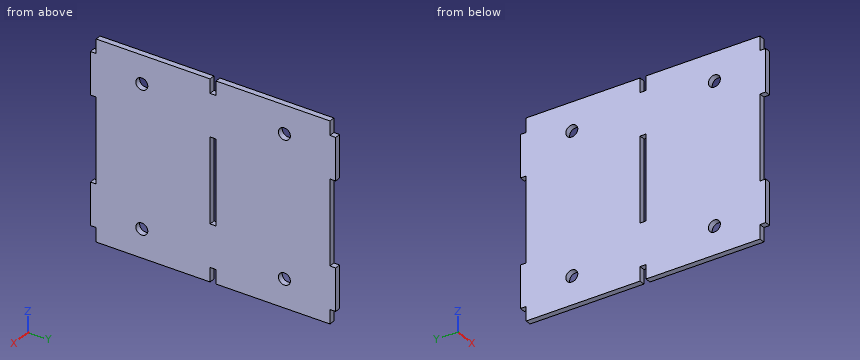
Autodesk Inventor part; units mm, degrees
ref_plane "YZ Plane" through (0, 0, 0) normal (1, 0, 0) x (0, 1, 0)
ref_plane "XZ Plane" through (0, 0, 0) normal (0, 1, 0) x (-1, 0, 0)
ref_plane "XY Plane" through (0, 0, 0) normal (0, 0, 1) x (1, 0, 0)
sketch "Sketch1" plane through (0, 0, 0) normal (1, 0, 0) x (0, 1, 0)
  line L0 (0, 15) -> (0, 0)
  line L1 (0, 15) -> (-2, 15)
  line L2 (-2, 15) -> (-2, 30)
  line L3 (-2, 30) -> (0, 30)
  line L4 (0, 30) -> (0, 35)
  line L5 (0, 35) -> (39.95, 35)
  line L6 (20, 0) -> (0, 0) construction
  line L7 (39.95, 35) -> (39.95, 30)
  line L8 (39.95, 30) -> (42.05, 30)
  line L9 (42.05, 15) -> (39.95, 15)
  line L10 (39.95, 15) -> (39.95, 0)
  line L11 (39.95, 0) -> (20, 0) construction
  line L12 (0, -15) -> (0, 0)
  line L13 (0, -15) -> (-2, -15)
  line L14 (-2, -15) -> (-2, -30)
  line L15 (-2, -30) -> (0, -30)
  line L16 (0, -30) -> (0, -35)
  line L17 (0, -35) -> (39.95, -35)
  line L18 (39.95, -35) -> (39.95, -30)
  line L19 (39.95, -30) -> (42.05, -30)
  line L20 (42.05, -15) -> (39.95, -15)
  line L21 (39.95, -15) -> (39.95, 0)
  line L22 (41, 30) -> (41, -30) construction
  line L23 (82, 15) -> (82, 0)
  line L24 (82, 15) -> (84, 15)
  line L25 (84, 30) -> (82, 30)
  line L26 (82, 30) -> (82, 35)
  line L27 (82, 35) -> (42.05, 35)
  line L28 (42.05, 35) -> (42.05, 30)
  line L29 (42.05, 15) -> (42.05, 0)
  line L30 (42.05, -35) -> (42.05, -30)
  line L31 (42.05, -15) -> (42.05, 0)
  line L32 (82, -15) -> (84, -15)
  line L33 (84, -15) -> (84, -30)
  line L34 (84, -30) -> (82, -30)
  line L35 (82, -30) -> (82, -35)
  line L36 (82, -15) -> (82, 0)
  line L37 (82, -35) -> (42.05, -35)
  line L38 (84, 30) -> (84, 15)
  dimension "d3" = 15
  dimension "d6" = 20
  dimension "d7" = 35
  dimension "d8" = 15
  dimension "d9" = 2
  dimension "d17" = 2.1
  dimension "d23" = 41
extrude "Wyciągnięcie proste1" add sketch "Sketch1" along normal blind 2
sketch "Szkic3" plane through (2, 0, 0) normal (1, 0, 0) x (0, 0, -1)
  line L0 (-25, 16) -> (25, 16) construction
  line L1 (25, 16) -> (25, 66) construction
  line L2 (25, 66) -> (-25, 66) construction
  line L3 (-25, 66) -> (-25, 16) construction
  line L4 (-25, 16) -> (25, 66) construction
  line L5 (25, 16) -> (-25, 66) construction
  line L6 (0, 41) -> (0, 42.05) construction
  line L7 (-15, 42.05) -> (15, 42.05) construction
  line L8 (0, 41) -> (15, 41) construction
  line L9 (15, 42.05) -> (15, 39.95) construction
  circle A0 centre (-25, 66) radius 2.1
  circle A1 centre (25, 66) radius 2.1
  circle A2 centre (25, 16) radius 2.1
  circle A3 centre (-25, 16) radius 2.1
  point P0 (0, 0)
  dimension "d18" = 4.2
  dimension "d19" = 50
  dimension "d20" = 50
extrude "Wyciągnięcie proste2" cut sketch "Szkic3" against normal up to surface (2 mm away)
sketch "Sketch4" plane through (2, 0, 0) normal (1, 0, 0) x (0, 0, -1)
  circle A0 centre (25, 16) radius 2.1
  circle A1 centre (-25, 16) radius 2.1
  circle A2 centre (25, 66) radius 2.1
  circle A3 centre (-25, 66) radius 2.1
  line L0 (-15, 42.05) -> (15, 42.05)
  line L1 (15, 42.05) -> (15, 39.95)
  line L2 (15, 39.95) -> (-15, 39.95)
  line L3 (-15, 39.95) -> (-15, 42.05)
  line L4 (-15, 0) -> (15, 0)
  line L5 (15, 0) -> (15, -2)
  line L6 (15, -2) -> (30, -2)
  line L7 (30, -2) -> (30, 0)
  line L8 (30, 0) -> (35, 0)
  line L9 (35, 0) -> (35, 39.95)
  line L10 (35, 39.95) -> (30, 39.95)
  line L11 (30, 39.95) -> (30, 42.05)
  line L12 (30, 42.05) -> (35, 42.05)
  line L13 (35, 42.05) -> (35, 82)
  line L14 (35, 82) -> (30, 82)
  line L15 (30, 82) -> (30, 84)
  line L16 (30, 84) -> (15, 84)
  line L17 (15, 84) -> (15, 82)
  line L18 (15, 82) -> (-15, 82)
  line L19 (-15, 82) -> (-15, 84)
  line L20 (-15, 84) -> (-30, 84)
  line L21 (-30, 84) -> (-30, 82)
  line L22 (-30, 82) -> (-35, 82)
  line L23 (-35, 82) -> (-35, 42.05)
  line L24 (-35, 42.05) -> (-30, 42.05)
  line L25 (-30, 42.05) -> (-30, 39.95)
  line L26 (-30, 39.95) -> (-35, 39.95)
  line L27 (-35, 39.95) -> (-35, 0)
  line L28 (-35, 0) -> (-30, 0)
  line L29 (-30, 0) -> (-30, -2)
  line L30 (-30, -2) -> (-15, -2)
  line L31 (-15, -2) -> (-15, 0)
  point P0 (0, 0)
equation "\"d6\" = 0.5 * d10"
properties part number "CH_01_0010_syringe_pump_servo" material "Aluminum 6061"
The listing builds one solid part. Answer for the finished solid, in the listing's coordinates (mm). Round coordinates to 2 decimals unless told otherwise and drop trailing zeros. Loops run counter-clockwise (first coordinate to the right, second up) from the corner with the lowest first, then second, coordinate; pieces in that order, holes last.
1) Given P1, Ø0.6, axis at x = 1, y = 41.5, coming from the -Z side; P2, Ø1, axis at x = 1, z = 32.5, coming from the -Y side; P3, Ø0.6, axis at x = 1, z = 33, coming from the +Y side, each flat-ended and moving along its own axis, determine where each tip first touches the part or whether it passes through.
Outcome:
P1: stops at z = -30
P2: stops at y = 0
P3: stops at y = 82
2) Consider line 1 (Y direction, x = 0.6, z = 25); line 2 (Z direction, x = 0.65, y = 41); line 3 (Z direction, x = 0.25, y = 65). Determine where each line is inside the solid, lowest interval first.
Outcome:
line 1: y = -2 to 13.9, 18.1 to 63.9, 68.1 to 84
line 2: z = -30 to -15, 15 to 30
line 3: z = -35 to -26.85, -23.15 to 23.15, 26.85 to 35
3) A cutting plane is placed at B-B on z = -25. Determine the outline of the cut face in (x, y), plus the area to 3 significant figures.
Outcome:
outline: (0, -2) - (2, -2) - (2, 13.9) - (0, 13.9) - close; (0, 18.1) - (2, 18.1) - (2, 63.9) - (0, 63.9) - close; (0, 68.1) - (2, 68.1) - (2, 84) - (0, 84) - close
area: 155 mm2
4) A cutting plane is placed at A-A on z = -7. Determine the outline of the cut face in (x, y).
Outcome:
outline: (0, 0) - (2, 0) - (2, 39.95) - (0, 39.95) - close; (0, 42.05) - (2, 42.05) - (2, 82) - (0, 82) - close
5) A cutting plane is placed at C-C on y = 66. Determine the outline of the cut face in (x, z).
Outcome:
outline: (0, -35) - (2, -35) - (2, -27.1) - (0, -27.1) - close; (0, -22.9) - (2, -22.9) - (2, 22.9) - (0, 22.9) - close; (0, 27.1) - (2, 27.1) - (2, 35) - (0, 35) - close
6) A cutting plane is placed at D-D on x = 1.35. Give the number of separate pieces and of enclosed holes in the cut face, plus the area to 3 significant figures.
Outcome:
separate pieces: 1
enclosed holes: 5
area: 5,720 mm2
